Work out the finished part from the listing and answer in its coordinate system (mm). A direction names the side the tool comes from. Give positions to 0.01 mm unless a question says otherwise; leave off trailing zeros. Write each loop counter-clockwise with the first axis right and the second up, starting at its lowest first coordinate (ties: lowest second). Pieces come first, ordered by that corner, then holes.
1) A tool of negligible diameter and unlimited length cuts with its end or side. For faces 1 (the face through (-75, 25, 42)), 2 (the face through (50, 87, 25.4)), 3 (the face through (-51, 25.4, 89)), from which of +Z, -Z, +X, -X, +Y, -Y can it reach the whole face along a straight path? Write none if from no direction.
2) Given pin 1 Ø12 at (x, y) = (35.5, 73.5) entering from +Z; pin 2 Ø1 at (x, y) = (45, 59.5) entering from -Z; pin 3 Ø6 at (x, y) = (-12, 92) entering from +Z; pin 4 Ø15 at (x, z) = (47, 71) entering from +Y, each flat-ended and moving along its own axis, determine where each tip first touches the part or whether it passes through.
3) Find section C-C (x = -45). Determine the outline of the cut face in (y, z).
4) Find section D-D (x = 12.5). Determine the outline of the cut face in (y, z), plus the area to 3 significant figures.
5) Find section A-A (y = 89). Determine the outline of the cut face in (x, z).
6) Find section B-B (z = 93). Determine the outline of the cut face in (x, y).
7) Straight lines are drawn through the part: probe 1 along Y at (x, z) = (-64, 100); probe 2 along X at (y, z) = (111, 34). For each, find the intervals that lie inside material, in ascending order.
```python
from build123d import *

# Parameters (mm, degrees)
BOSS_EXTRUDE1_DEPTH      = 75
BOSS_EXTRUDE1_DEPTH_BACK = 75
BOSS_EXTRUDE2_DEPTH      = 25.4
BOSS_EXTRUDE2_DEPTH_BACK = 25.4


with BuildPart() as part:
    # Sketch1 → Boss-Extrude1 (new, two sides: drawn at the far end of the back side and taken through both)
    with BuildSketch(Plane.YZ.offset(-BOSS_EXTRUDE1_DEPTH_BACK)):
        Polygon((0, 0), (0, 150), (25.4, 150), (25.4, 25.4), (150, 25.4), (150, 0), align=None)
    extrude(amount=BOSS_EXTRUDE1_DEPTH + BOSS_EXTRUDE1_DEPTH_BACK)

    # Sketch3 → Boss-Extrude2 (add, two sides: drawn at the far end of the back side and taken through both)
    with BuildSketch(Plane.YZ.offset(-BOSS_EXTRUDE2_DEPTH_BACK)):
        Polygon((0, 150), (25.4, 150), (150, 25.4), (150, 0), (0, 0), align=None)
    extrude(amount=BOSS_EXTRUDE2_DEPTH + BOSS_EXTRUDE2_DEPTH_BACK)


solid = part.part
```
Results:
1. face 1: +Z, -Z, -X, +Y, -Y
1. face 2: +Z, +X, +Y
1. face 3: +Z, -X, +Y
2. pin 1: stops at z = 25.4
2. pin 2: stops at z = 0
2. pin 3: stops at z = 86.4
2. pin 4: stops at y = 25.4
3. outline: (0, 0) - (150, 0) - (150, 25.4) - (25.4, 25.4) - (25.4, 150) - (0, 150) - close
4. outline: (0, 0) - (150, 0) - (150, 25.4) - (25.4, 150) - (0, 150) - close
4. area: 14,700 mm2
5. outline: (-75, 0) - (75, 0) - (75, 25.4) - (25.4, 25.4) - (25.4, 86.4) - (-25.4, 86.4) - (-25.4, 25.4) - (-75, 25.4) - close
6. outline: (-75, 0) - (75, 0) - (75, 25.4) - (25.4, 25.4) - (25.4, 82.4) - (-25.4, 82.4) - (-25.4, 25.4) - (-75, 25.4) - close
7. probe 1: y = 0 to 25.4
7. probe 2: x = -25.4 to 25.4
